Read the model definition and answer for the solid it produces. Units are mm, in the model's axes. Face numbers are marked on the shaded views. A direction names the side the tool comes from. Give positions to 0.01 mm unless a question says otherwise; leave off trailing zeros. Order: outer loops, then holes, each group sorted by start corner. A loop starts at its lowest first (then second) coordinate and runs counter-clockwise, first axis right, second up. Notation, with made-up numbers: (86, 70.5) -> (115, 70.5) arc R20 ccw to (115, 102.5) -> close; hole circle Ø3 at (88.25, 9). An arc over 180 degrees is marked (long way). Use one line per item in the form item = value.
```python
from build123d import *

# Parameters (mm, degrees)
SKETCH1_R           = 12.7
BOSS_EXTRUDE1_DEPTH = 30.1625
SKETCH4_R           = 25.4
BOSS_EXTRUDE2_DEPTH = 50.8
CUT_EXTRUDE1_DEPTH  = 11.176
SKETCH3_R           = 6
CUT_EXTRUDE2_DEPTH  = 8
SKETCH5_R           = 3.175
BOSS_EXTRUDE3_DEPTH = 6.604
CUT_EXTRUDE3_START  = -6.35
SKETCH9_R           = 25.4
SKETCH9_R_2         = 6.35
CUT_EXTRUDE3_DEPTH  = 38.1
FILLET1_R           = 3.175
CHAMFER1_SIZE       = 1.27


with BuildPart() as part:
    # Sketch1 → Boss-Extrude1 (new body)
    with BuildSketch(Plane(origin=(0, 0, 0), x_dir=(1, 0, 0), z_dir=(0, 1, 0))):
        Circle(SKETCH1_R)
    extrude(amount=BOSS_EXTRUDE1_DEPTH)

    # Sketch4 → Boss-Extrude2 (add)
    with BuildSketch(Plane(origin=(0, 30.1625, 0), x_dir=(1, 0, 0), z_dir=(0, 1, 0))):
        Circle(SKETCH4_R)
    extrude(amount=BOSS_EXTRUDE2_DEPTH)

    # Sketch2 → Cut-Extrude1 (cut)
    with BuildSketch(Plane.XZ):
        with BuildLine():
            Line((-7, 2.899494937), (-8.776962921, 1.122532015))
            ThreePointArc((-8.776962921, 1.122532015), (-9.241930906, 0), (-8.776962921, -1.122532015))
            Line((-8.776962921, -1.122532015), (-7, -2.899494937))
            Line((-7, -2.899494937), (-7, 2.899494937))
        make_face()
        Polygon((-2.899494937, 7), (-7, 2.899494937), (-7, -2.899494937), (-2.899494937, -7), (2.899494937, -7), (7, -2.899494937), (7, 2.899494937), (2.899494937, 7), align=None)
        with BuildLine():
            Line((-7, 5.4125), (-7, 2.899494937))
            Line((-7, 2.899494937), (-2.899494937, 7))
            Line((-2.899494937, 7), (-5.4125, 7))
            ThreePointArc((-5.4125, 7), (-6.535032015, 6.535032015), (-7, 5.4125))
        make_face()
        with BuildLine():
            Line((-1.122532015, 8.776962921), (-2.899494937, 7))
            Line((-2.899494937, 7), (2.899494937, 7))
            Line((2.899494937, 7), (1.122532015, 8.776962921))
            ThreePointArc((1.122532015, 8.776962921), (0, 9.241930906), (-1.122532015, 8.776962921))
        make_face()
        with BuildLine():
            Line((5.4125, 7), (2.899494937, 7))
            Line((2.899494937, 7), (7, 2.899494937))
            Line((7, 2.899494937), (7, 5.4125))
            ThreePointArc((7, 5.4125), (6.535032015, 6.535032015), (5.4125, 7))
        make_face()
        with BuildLine():
            Line((8.776962921, 1.122532015), (7, 2.899494937))
            Line((7, 2.899494937), (7, -2.899494937))
            Line((7, -2.899494937), (8.776962921, -1.122532015))
            ThreePointArc((8.776962921, -1.122532015), (9.241930906, 0), (8.776962921, 1.122532015))
        make_face()
        with BuildLine():
            Line((7, -2.899494937), (2.899494937, -7))
            Line((2.899494937, -7), (5.4125, -7))
            ThreePointArc((5.4125, -7), (6.535032015, -6.535032015), (7, -5.4125))
            Line((7, -5.4125), (7, -2.899494937))
        make_face()
        with BuildLine():
            Line((2.899494937, -7), (-2.899494937, -7))
            Line((-2.899494937, -7), (-1.122532015, -8.776962921))
            ThreePointArc((-1.122532015, -8.776962921), (0, -9.241930906), (1.122532015, -8.776962921))
            Line((1.122532015, -8.776962921), (2.899494937, -7))
        make_face()
        with BuildLine():
            Line((-2.899494937, -7), (-7, -2.899494937))
            Line((-7, -2.899494937), (-7, -5.4125))
            ThreePointArc((-7, -5.4125), (-6.535032015, -6.535032015), (-5.4125, -7))
            Line((-5.4125, -7), (-2.899494937, -7))
        make_face()
    extrude(amount=-CUT_EXTRUDE1_DEPTH, mode=Mode.SUBTRACT)

    # Sketch3 → Cut-Extrude2 (cut)
    with BuildSketch(Plane.XZ.offset(-11.176)):
        Circle(SKETCH3_R)
    extrude(amount=-CUT_EXTRUDE2_DEPTH, mode=Mode.SUBTRACT)

    # Sketch5 → Boss-Extrude3 (add)
    with BuildSketch(Plane(origin=(0, 80.9625, 0), x_dir=(1, 0, 0), z_dir=(0, 1, 0))):
        Circle(SKETCH5_R)
    extrude(amount=BOSS_EXTRUDE3_DEPTH)

    # Sketch9 → Cut-Extrude3 (cut)
    with BuildSketch(Plane(origin=(0, 80.9625, 0), x_dir=(1, 0, 0), z_dir=(0, 1, 0)).offset(CUT_EXTRUDE3_START)):
        Circle(SKETCH9_R)
        Circle(SKETCH9_R_2, mode=Mode.SUBTRACT)
    extrude(amount=-CUT_EXTRUDE3_DEPTH, mode=Mode.SUBTRACT)

    # Fillet1
    fillet1_edges = [part.edges().sort_by_distance(p)[0] for p in [
        (-6.35, 36.5125, 0),
        (-6.35, 74.6125, 0),
    ]]
    fillet(fillet1_edges, radius=FILLET1_R)

    # Chamfer1
    chamfer1_edges = [part.edges().sort_by_distance(p)[0] for p in [
        (-25.4, 80.9625, 0),
        (-25.4, 36.5125, 0),
    ]]
    chamfer(chamfer1_edges, length=CHAMFER1_SIZE)


solid = part.part
```
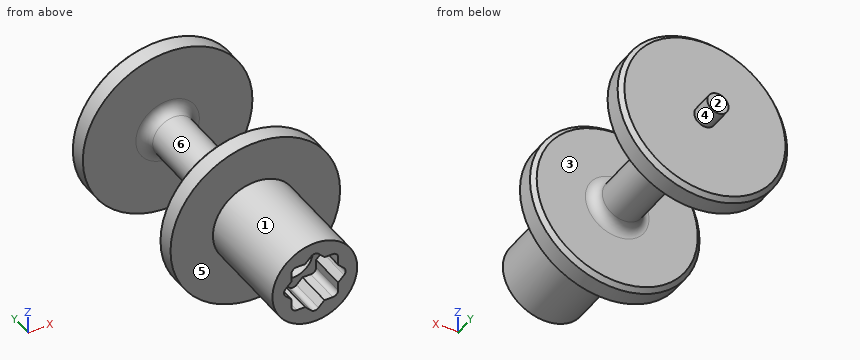
Item 1: Given pin 1 Ø1 at (x, z) = (12, 6.5) entering from +Y; pin 2 Ø1.3 at (y, z) = (7.5, -4) entering from -X; pin 3 Ø12 at (x, y) = (16, 13) entering from +Z, each flat-ended and moving along its own axis, determine where each tip first touches the part or whether it passes through.
Checks:
pin_1 = 80.96
pin_2 = -12.25
pin_3 = 7.83
Item 2: Straight lines are drawn through the part: L1, parallel to Y at x = 22, z = 3.5; L2, parallel to Z at x = 0, y = 13.75; L3, parallel to Y at x = 1, z = -11.5. For each, find the intervals that lie inside material, in ascending order. Write a range as from..to.
Checks:
L1 = 30.16..36.51, 74.61..80.96
L2 = -12.7..-6, 6..12.7
L3 = 0..36.51, 74.61..80.96
Item 3: The part is cut by section B-B on y = 57. Give the vertices of the cut face in (x, z), and give its area (3 significant figures).
Checks:
outline = circle Ø12.7 at (0, 0)
area = 127 mm²
Item 4: Which of the six approach directions +Z, -Z, +X, -X, +Y, -Y give full straight-line access (tool end or side, diameter ignored) to the marked faces 4, 5 and 6?
Checks:
face_4 = +Y
face_5 = -Y
face_6 = none
Item 5: Determine the mould class of the marked faces 1, 2 and 3 for opening direction Y: +Y half, -Y half, draft (parallel to the pull), parting line (faces both ways), or undercut.
Checks:
face_1 = draft
face_2 = +Y half
face_3 = undercut
Item 6: The part is cut by section A-A on y = 26.5. Give the vertices of the cut face in (x, z), and give its area (3 significant figures).
Checks:
outline = circle Ø25.4 at (0, 0)
area = 507 mm²
